The listing builds one solid part. Answer for the finished solid, in the listing's coordinates (mm). Give positions to 0.01 mm unless a question says otherwise; leave off trailing zeros. Loops run counter-clockwise (first coordinate to the right, second up) from the corner with the lowest first, then second, coordinate; pieces in that order, holes last. Notation, with made-up numbers: (39.25, 10) - (91.25, 10) arc R15 ccw to (91.25, 19) - close; hole circle Ø1 at (85.25, 20.25). An arc over 180 degrees is marked (long way). Write each question's results on one line, items separated by ' | '.
from build123d import *

# Parameters (mm, degrees)
F1_DEPTH = 2.5
F2_R     = 2.75
F3_DEPTH = 2.5


# Not quite as in the source:
# - a pattern or mirror of a feature is missing from the dataset's text; its kind, count and spacing are read off the source's solid


with BuildPart() as f1:
    # F0 (on Top) → F1 (new body, symmetric)
    with BuildSketch(Plane.XY):
        with BuildLine():
            Line((3.853342479, 2.6833219012), (2.7102889432, 4.112138821))
            Line((2.7102889432, 4.112138821), (-4.6141804357, 1.7322744554))
            ThreePointArc((-4.6141804357, 1.7322744554), (-9.5, 0), (-4.6141804357, -1.7322744554))
            Line((-4.6141804357, -1.7322744554), (2.7102889432, -4.112138821))
            Line((2.7102889432, -4.112138821), (3.853342479, -2.6833219012))
            Line((3.853342479, -2.6833219012), (3.853342479, -2.6829979227))
            ThreePointArc((3.853342479, -2.6829979227), (0.5, 0), (3.853342479, 2.6829979227))
            Line((3.853342479, 2.6829979227), (3.853342479, 2.6833219012))
        make_face()
    extrude(amount=F1_DEPTH, both=True)

    # F2 (on face) → F3 (join)
    with BuildSketch(Plane.XY.offset(2.5)):
        with Locations((-6.75, 0)):
            Circle(F2_R)
    f3 = extrude(amount=F3_DEPTH)

    # F3_copies: F3 across plane
    add(f3.mirror(Plane(origin=(0, 0, 0), x_dir=(-1, 0, 0), z_dir=(0, 0, -1))))


solid = f1.part
Item 1: A cutting plane is placed at C-C, the plane y = 2.5. Determine the outline of the cut face in (x, z).
Values found:
outline: (-7.9, -5) - (-5.6, -5) - (-5.6, 5) - (-7.9, 5) - close; (-2.25, -2.5) - (2.1, -2.5) - (2.1, 2.5) - (-2.25, 2.5) - close
Item 2: For a pull along X with two mould halves and no side action, classify faces 1 (the face through (-1.003, -2.906, 0.035)), 2 (the face through (3.29, 3.39, 0.04)), 3 (the face through (-7, 0, 5)), 4 (the face through (-0.9, 2.94, 0.04)) as released by +X, released by -X, zero draft, split by the parting line, or undercut.
Values found:
face 1: undercut | face 2: released by +X | face 3: zero draft | face 4: undercut
Item 3: A cutting plane is placed at A-A, the plane y = 0. Determine the outline of the cut face in (x, z), plus the area to 3 significant figures.
Values found:
outline: (-9.5, -5) - (-4, -5) - (-4, -2.5) - (0.5, -2.5) - (0.5, 2.5) - (-4, 2.5) - (-4, 5) - (-9.5, 5) - close | area: 77.5 mm²
Item 4: A cutting plane is placed at D-D, the plane x = 3.25. Determine the outline of the cut face in (y, z).
Values found:
outline: (-3.44, -2.5) - (-2.75, -2.5) - (-2.75, 2.5) - (-3.44, 2.5) - close; (2.75, -2.5) - (3.44, -2.5) - (3.44, 2.5) - (2.75, 2.5) - close
Item 5: A cutting plane is placed at B-B, the plane x = -6.75. Determine the outline of the cut face in (y, z), plus the area to 3 significant figures.
Values found:
outline: (-2.75, -5) - (2.75, -5) - (2.75, 5) - (-2.75, 5) - close | area: 55.0 mm²
Item 6: Find the intervals of material crossed by line 1 along Z through (x, y) = (-1.5, 1); line 2 along X through (y, z) = (0, -0.35); line 3 along Y through (x, z) = (3.25, -1.1), in increasing order. Write a range as [from, to].
Values found:
line 1: z = [-2.5, 2.5] | line 2: x = [-9.5, 0.5] | line 3: y = [-3.44, -2.75], [2.75, 3.44]
Item 7: Flat-ended cylindrical pins translate along their axes: P1, Ø5, axis at x = 2, z = 2, coming from the -Y side; P2, Ø3, axis at x = -1, y = -2.5, coming from the +Z side; P3, Ø6, axis at x = -1, z = 1.5, coming from the +Y side; P4, Ø6, axis at x = -4, z = 1.5, coming from the +Y side. Find the tip coordinate at first contact, or state that the pin passes through.
Values found:
P1: stops at y = -4.11 | P2: stops at z = 2.5 | P3: stops at y = 3.88 | P4: stops at y = 2.91
